```python
from build123d import *

# Parameters (mm, degrees)
CROQUIS1_R              = 3
SALIENTE_EXTRUIR1_DEPTH = 5
REDONDEO7_R             = 4


with BuildPart() as part:
    # Croquis1 → Saliente-Extruir1 (new, symmetric)
    with BuildSketch(Plane(origin=(0, 0, 0), x_dir=(-1, 0, 0), z_dir=(0, 1, 0))):
        with BuildLine():
            Line((52.388821078, 22.035902101), (260.523173553, 7.481730377))
            ThreePointArc((260.523173553, 7.481730377), (267.481730377, -0.523173553), (259.476826447, -7.481730377))
            Line((259.476826447, -7.481730377), (51.342473972, 7.072441348))
            ThreePointArc((51.342473972, 7.072441348), (26.697288319, 4.552818898), (4.339230902, -6.117276778))
            ThreePointArc((4.339230902, -6.117276778), (-6.117276778, -4.339230902), (-4.339230902, 6.117276778))
            ThreePointArc((-4.339230902, 6.117276778), (22.644631497, 18.994978455), (52.388821078, 22.035902101))
        make_face()
        with Locations(Location((0, 0, 0), (0, 0, 90))):
            Circle(CROQUIS1_R, mode=Mode.SUBTRACT)
        with Locations(Location((260, 0, 0), (0, 0, 90))):
            Circle(CROQUIS1_R, mode=Mode.SUBTRACT)
    extrude(amount=SALIENTE_EXTRUIR1_DEPTH, both=True)

    # Redondeo7
    redondeo7_edges = [part.edges().sort_by_distance(p)[0] for p in [
        (-155.409650209, 5, -0.204644515),
        (-267.481730377, 5, -0.523173553),
        (-156.455997315, 5, 14.758816239),
        (-22.644631497, 5, 18.994978455),
        (6.117276778, 5, -4.339230902),
        (-22.644631497, -5, 18.994978455),
        (-156.455997315, -5, 14.758816239),
        (-267.481730377, -5, -0.523173553),
        (-155.409650209, -5, -0.204644515),
        (-26.697288319, -5, 4.552818898),
        (6.117276778, -5, -4.339230902),
        (-26.697288319, 5, 4.552818898),
    ]]
    fillet(redondeo7_edges, radius=REDONDEO7_R)


solid = part.part
```
Can you work these out from the model? Positions are in its coordinate system, mm. A direction names the side the tool comes from. Coordinates: 2 decimals unless noted, no trailing zeros. Answer as a JSON object with one key per item and string values.
1) If I drill on line 1 (Z direction, x = -260, y = 0.75); line 2 (Z direction, x = -168, y = -4.25); line 3 (Z direction, x = -193, y = -4.5), over which ranges is the centre line in solid material (lowest first)?
Results:
{"line 1": "z = -7.5 to -3, 3 to 7.52", "line 2": "z = 0.59 to 12.28", "line 3": "z = -0.76 to 10.13"}
2) Thinking about a two-plate mould opening in Z: for faces 1 (the face through (-155, 0.01, 14.86)), 2 (the face through (0.9, -0.07, 2.86)), 3 (the face through (-154.04, -3.86, 1.1)), which applies, pulls with the +Z half, pulls with the -Z half, needs draft (parallel to the pull), parting line crosses it, or undercut?
Results:
{"face 1": "pulls with the +Z half", "face 2": "undercut", "face 3": "pulls with the -Z half"}
3) Imagine slicing it at A-A (z = 0). Count the separate pieces of the cut face and the enclosed holes in it, then the cut area to 3 significant figures.
Results:
{"separate pieces": "4", "enclosed holes": "0", "area": "1,120 mm^2"}
4) For P1, Ø2, axis at x = -147, y = -1, coming from the +Z side; P2, Ø3, axis at x = -100, y = -3, coming from the +Z side; P3, Ø1, axis at y = 2.5, z = 2.5, coming from the +X side, each with a flat end and sliding along its axis, tell me the tip position at first contact or that it passes through.
Results:
{"P1": "stops at z = 15.49", "P2": "stops at z = 18.7", "P3": "stops at x = 7.01"}
5) For faces 4 (the face through (-27.033, 0.014, 4.646)), 5 (the face through (-154.04, 3.86, 1.1)), 6 (the face through (-257, 0, 0)), which set-ups out of +Z, -Z, +X, -X, +Y, -Y let a thin tool reach every point of the face, with its end or its side?
Results:
{"face 4": "-Z, +Y, -Y", "face 5": "-Z, +Y", "face 6": "+Y, -Y"}
